from build123d import *

# Parameters (mm, degrees)
SKETCH1_R           = 20.32
BOSS_EXTRUDE1_DEPTH = 21.59
SKETCH2_W           = 15.24
SKETCH2_H           = 4.318
CUT_EXTRUDE1_REACH  = 37.943
SKETCH4_R           = 1.27
CIRPATTERN1_COUNT   = 6
SKETCH9_R           = 1.905
CUT_EXTRUDE3_DEPTH  = 51.305467894
SKETCH10_R          = 7.112
CUT_EXTRUDE8_DEPTH  = 17.272


with BuildPart() as part:
    # Sketch1 → Boss-Extrude1 (new body)
    with BuildSketch(Plane(origin=(0, 0, 0), x_dir=(1, 0, 0), z_dir=(0, 1, 0))):
        with Locations(Location((0, 0, 0), (0, 0, 270))):
            Circle(SKETCH1_R)
    extrude(amount=BOSS_EXTRUDE1_DEPTH)

    # Sketch2 → Cut-Revolve1 (revolve, cut)
    with BuildSketch(Plane.XY, mode=Mode.PRIVATE) as cut_revolve1_sk:
        with Locations((-7.62, 19.431)):
            Rectangle(SKETCH2_W, SKETCH2_H)
    revolve(cut_revolve1_sk.sketch.rotate(Axis((0, 22.78347084, 0), (0, -1, 0)), 270), axis=Axis((0, 22.78347084, 0), (0, -1, 0)), mode=Mode.SUBTRACT)

    # Sketch4 → Cut-Extrude1 (cut, up to next)
    with BuildSketch(Plane(origin=(0, 21.59, 0), x_dir=(1, 0, 0), z_dir=(0, 1, 0)), mode=Mode.PRIVATE) as cut_extrude1_sk1:
        with Locations(Location((0, 17.78, 0), (0, 0, 270))):
            Circle(SKETCH4_R)
    cut_extrude1_tool1 = extrude(cut_extrude1_sk1.sketch, amount=-CUT_EXTRUDE1_REACH, mode=Mode.PRIVATE) & part.part
    cut_extrude1 = cut_extrude1_tool1.solids().sort_by_distance((0, 21.59, -17.78))[0]
    add(cut_extrude1, mode=Mode.SUBTRACT)

    # CirPattern1: Cut-Extrude1 ×6 about axis
    cirpattern1_axis = Axis((0, 0, 0), (0, 1, 0))
    for i in range(1, CIRPATTERN1_COUNT):
        add(cut_extrude1.rotate(cirpattern1_axis, i * 360 / CIRPATTERN1_COUNT), mode=Mode.SUBTRACT)

    # Sketch8 → Cut-Revolve4 (revolve, cut)
    with BuildSketch(Plane.XY, mode=Mode.PRIVATE) as cut_revolve4_sk:
        Polygon((-4.699, 17.272), (-13.97, 17.272), (-13.97, 16.002), (-4.699, 6.731), align=None)
    revolve(cut_revolve4_sk.sketch.rotate(Axis((0, 22.78347084, 0), (0, -1, 0)), 270), axis=Axis((0, 22.78347084, 0), (0, -1, 0)), mode=Mode.SUBTRACT)

    # Sketch9 → Cut-Extrude3 (cut, through all)
    with BuildSketch(Plane(origin=(20.32, 0, 0), x_dir=(0, 0, -1), z_dir=(1, 0, 0))):
        with Locations((0, 21.59)):
            Circle(SKETCH9_R)
    extrude(amount=-CUT_EXTRUDE3_DEPTH, mode=Mode.SUBTRACT)

    # Sketch10 → Cut-Extrude8 (cut)
    with BuildSketch(Plane(origin=(0, 0, 0), x_dir=(1, 0, 0), z_dir=(0, 1, 0))):
        with Locations(Location((0, 0, 0), (0, 0, 270))):
            Circle(SKETCH10_R)
    extrude(amount=CUT_EXTRUDE8_DEPTH, mode=Mode.SUBTRACT)


solid = part.part
Geometry: final body of the model. Coordinates: model frame, mm. A direction names the side the tool comes from. Give positions to 0.01 mm unless a question says otherwise; leave off trailing zeros. Loops run counter-clockwise (first coordinate to the right, second up) from the corner with the lowest first, then second, coordinate; pieces in that order, holes last. Notation, with made-up numbers: M 81,87 L 93,87 A25 ccw 93,100 Z; hole C -33,86 d7. An arc over 180 degrees is marked long. Put each result on its own line as item: value. Start each with the question number.
1) Access query for faces 5 (the flat face through (4.4, 17.272, 13.5)), 6 (the flat face through (-9, 0, 0)). Directions: +Z, -Z, +X, -X, +Y, -Y. A direction counts if a zero-diameter tool reaches every point of the face in a straight line with its end or side. Return the directions, or none.
2) Pull-direction query (X, two-part tool) for faces 1 (the cylindrical face through (-0.06, 10.95, 19.05)), 2 (the cylindrical face through (20.147, 10.644, -2.645)), 3 (the conical face through (-2.236, 9.477, 7.101)), 4 (the cylindrical face through (17.757, 19.685, 0.042)); classes: pulls with the +X half, pulls with the -X half, needs draft (parallel to the pull), parting line crosses it, or undercut.
3) Contact query for flat-ended pins moving along their axis: pin 1 (1.5 mm diameter, centred on x = -1, z = -12.5, fed in from +Y); pin 2 (1 mm diameter, centred on x = 13, y = 11.5, fed in from -Z); pin 3 (5 mm diameter, centred on x = 12.5, y = 17.5, fed in from -Z); pin 4 (1.5 mm diameter, centred on x = 0, z = 17.78, fed in from -Y). Output: stop coordinate, or through.
4) Cut plane A-A (z = 0). Output: boundary loops of the cut face in (x, y) (3 decimals).
5) Cut plane D-D (z = -8.89). Give the number of separate pieces and of enclosed holes in the cut face, then the cut area to 3 significant figures.
6) Ray query, line 1 along X through (y, z) = (16.25, -8.89); line 2 along X through (y, z) = (2, -8.5); line 3 along X through (y, z) = (6, 0). Return the intervals inside material, ascending.
7) Cut plane B-B (x = 0). Output: boundary loops of the cut face in (y, z).
8) Cut plane C-C (y = 18). Output: boundary loops of the cut face in (x, z) (3 decimals).
Verdict:
1. face 5: +Y
1. face 6: +Z, -Z, +X, -X, -Y
2. face 1: undercut
2. face 2: parting line crosses it
2. face 3: undercut
2. face 4: needs draft
3. pin 1: y = 15.32
3. pin 2: z = -16.02
3. pin 3: z = -17.69
3. pin 4: through
4. outline: M -20.32,0 L -7.112,0 L -7.112,9.144 L -13.97,16.002 L -13.97,17.272 L -15.24,17.272 L -15.24,19.685 L -20.32,19.685 Z; M 7.112,0 L 20.32,0 L 20.32,19.685 L 15.24,19.685 L 15.24,17.272 L 13.97,17.272 L 13.97,16.002 L 7.112,9.144 Z
5. separate pieces: 3
5. enclosed holes: 0
5. area: 475 mm2
6. line 1: -18.27 to -16.67, -14.13 to -10.78, 10.78 to 14.13, 16.67 to 18.27
6. line 2: -18.46 to -16.61, -14.19 to 14.19, 16.61 to 18.46
6. line 3: -20.32 to -7.11, 7.11 to 20.32
7. outline: M 0,-20.32 L 21.59,-20.32 L 21.59,-19.05 L 0,-19.05 Z; M 0,-16.51 L 21.59,-16.51 L 21.59,-15.24 L 17.27,-15.24 L 17.27,-13.97 L 16,-13.97 L 9.14,-7.11 L 0,-7.11 Z; M 0,7.11 L 9.14,7.11 L 16,13.97 L 17.27,13.97 L 17.27,15.24 L 21.59,15.24 L 21.59,16.51 L 0,16.51 Z; M 0,19.05 L 21.59,19.05 L 21.59,20.32 L 0,20.32 Z
8. outline: C 0,0 d40.64; hole C -15.398,-8.89 d2.54; hole C -15.398,8.89 d2.54; hole C 0,0 d30.48; hole C 0,-17.78 d2.54; hole C 0,17.78 d2.54; hole C 15.398,-8.89 d2.54; hole C 15.398,8.89 d2.54
